from build123d import *

# Parameters (mm, degrees)
F0_R      = 34.925
F0_R_2    = 1.5875
F1_DEPTH  = 6.35
F2_R      = 22.5
F3_DEPTH  = 3.175
F4_R      = 19.685
F5_DEPTH  = 3.176
F6_R      = 23.495
F6_R_2    = 19.685
F7_DEPTH  = 19.05
F8_R      = 23.495
F9_DEPTH  = 6.35
F10_R     = 12.5
F11_DEPTH = 127
F12_R     = 15.24
F13_DEPTH = 1.27
F14_W     = 46.99
F14_H     = 20.32
F15_DEPTH = 25.4


with BuildPart() as f1:
    # F0 (on Top) → F1 (new body)
    with BuildSketch(Plane.XY):
        Circle(F0_R)
        with Locations((-16.42272, -22.603935)):
            Circle(F0_R_2, mode=Mode.SUBTRACT)
        with Locations((16.42272, -22.603935)):
            Circle(F0_R_2, mode=Mode.SUBTRACT)
        with Locations((-26.572519, 8.633935)):
            Circle(F0_R_2, mode=Mode.SUBTRACT)
        with Locations((26.572519, 8.633935)):
            Circle(F0_R_2, mode=Mode.SUBTRACT)
        with Locations((0, 27.94)):
            Circle(F0_R_2, mode=Mode.SUBTRACT)
    extrude(amount=F1_DEPTH)

    # F2 (on face) → F3 (cut)
    with BuildSketch(Plane(origin=(0, 0, 0), x_dir=(1, 0, 0), z_dir=(0, 0, -1))):
        Circle(F2_R)
    extrude(amount=-F3_DEPTH, mode=Mode.SUBTRACT)

    # F4 (on face) → F5 (cut, through all)
    with BuildSketch(Plane(origin=(0, 0, 3.175), x_dir=(1, 0, 0), z_dir=(0, 0, -1))):
        Circle(F4_R)
    extrude(amount=-F5_DEPTH, mode=Mode.SUBTRACT)

    # F6 (on face) → F7 (join)
    with BuildSketch(Plane.XY.offset(6.35)):
        Circle(F6_R)
        Circle(F6_R_2, mode=Mode.SUBTRACT)
    extrude(amount=F7_DEPTH)

    # F8 (on face) → F9 (join)
    with BuildSketch(Plane.XY.offset(25.4)):
        Circle(F8_R)
    extrude(amount=F9_DEPTH)

    # F10 (on face) → F11 (join)
    with BuildSketch(Plane.XY.offset(31.75)):
        Circle(F10_R)
    extrude(amount=F11_DEPTH)

    # F12 (on face) → F13 (join)
    with BuildSketch(Plane.XY.offset(31.75)):
        Circle(F12_R)
    extrude(amount=F13_DEPTH)

    # F14 (on Front) → F15 (cut)
    with BuildSketch(Plane.XZ):
        with Locations((0, 19.05)):
            Rectangle(F14_W, F14_H)
    extrude(amount=-F15_DEPTH, mode=Mode.SUBTRACT)


solid = f1.part
For this review, take the finished solid that the model builds, in its own axes (mm). A direction names the side the tool comes from. Round coordinates to 2 decimals unless told otherwise and drop trailing zeros. Write each loop counter-clockwise with the first axis right and the second up, starting at its lowest first coordinate (ties: lowest second). Pieces come first, ordered by that corner, then holes. Notation, with made-up numbers: M 15.25,-38 L 47.25,-38 A26 cw 47.25,-9 Z; hole C 68,41 d6. An arc over 180 degrees is marked long. Write item = value, one per line. Start each with the question number.
(1) We need section A-A (x = 0). Give the number of separate pieces and of enclosed holes in the cut face, then the cut area to 3 significant figures.
(2) We need section D-D (z = 79). Give the boundary of the cut face in (x, y).
(3) The part is to be moulded in two halves that separate along Y. For faces 1 (the face through (0, 24, 6.35)), 2 (the face through (10.382, 19.961, 1.565)), 3 (the face through (-5.093, -22.936, 18.872)), 4 (the face through (0, 0, 26)), say which applies: +Y half, -Y half, draft (parallel to the pull), parting line (faces both ways), or undercut.
(4) For faces 5 (the face through (-3.3, -14.88, 32.38)), 6 (the face through (0, -8, 25.4)), 7 (the face through (0, 20, 3.175)), list the 3-axis set-ups (+Z, -Z, +X, -X, +Y, -Y) from which the entire face can be reached by the end or side of a thin tool; tool diameter is ignored.
(5) We need section C-C (y = -1.5). Give the boundary of the cut face in (x, z) (3 decimals).
(6) For line 1 along Z through (x, y) = (19.5, 12); line 2 along Z through (x, y) = (-29, 11.5); line 3 along Z through (x, y) = (14.5, -8), list the stretches that pass through material, from the lowest coordinate up.
(7) Clearance check with flat-ended pins moving along their axes: pin 1 Ø7 at (x, y) = (-1, 10.5) entering from -Z; pin 2 Ø5 at (x, y) = (9.5, -23) entering from +Z; pin 3 Ø12 at (x, y) = (15.5, 5) entering from -Z (3 decimals). State where each tip first meets the part, or that it passes through.
Results found:
q1.separate_pieces = 3
q1.enclosed_holes = 0
q1.area = 3,630 mm²
q2.outline = C 0,0 d25
q3.face_1 = draft
q3.face_2 = undercut
q3.face_3 = parting line
q3.face_4 = +Y half
q4.face_5 = +Z
q4.face_6 = -Z, +Y
q4.face_7 = -Z
q5.outline = M -34.893,0 L -22.45,0 L -22.45,3.175 L -19.628,3.175 L -19.628,25.4 L 19.628,25.4 L 19.628,3.175 L 22.45,3.175 L 22.45,0 L 34.893,0 L 34.893,6.35 L 23.447,6.35 L 23.447,31.75 L 15.166,31.75 L 15.166,33.02 L 12.41,33.02 L 12.41,158.75 L -12.41,158.75 L -12.41,33.02 L -15.166,33.02 L -15.166,31.75 L -23.447,31.75 L -23.447,6.35 L -34.893,6.35 Z
q6.line_1 = 0 to 8.89, 29.21 to 31.75
q6.line_2 = 0 to 6.35
q6.line_3 = 25.4 to 31.75
q7.pin_1 = 29.21
q7.pin_2 = 31.75
q7.pin_3 = 3.175
